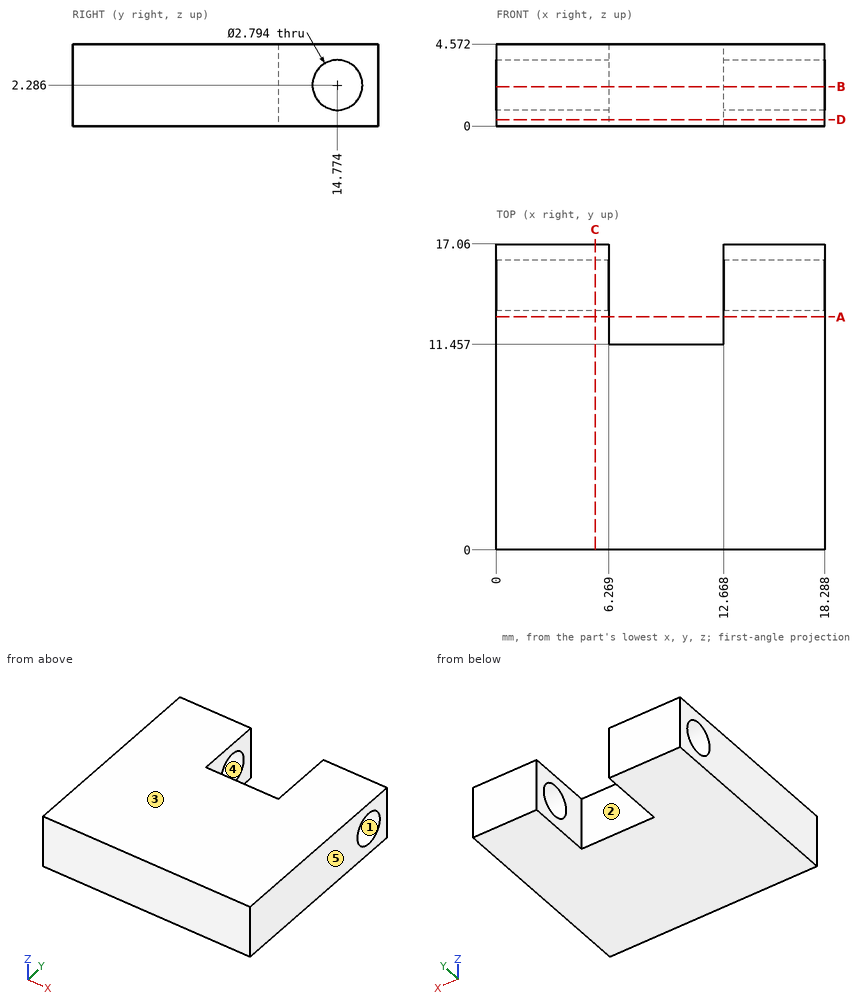
Check sheet for the drawn part. Datum: minimum x, y, z corner. Units: mm. A direction names the side the tool comes from. Coordinates: 2 decimals unless noted, no trailing zeros. Order: outer loops, then holes, each group sorted by start corner. A loop starts at its lowest first (then second) coordinate and runs counter-clockwise, first axis right, second up. Notation, with made-up numbers: (80, -32.75) -> (113, -32.75) arc R22 cw to (113, -5.75) -> close; hole circle Ø11 at (58.5, 29). An arc over 180 degrees is marked (long way). Use a Markdown table: item, result. Add a question column.
1. Cross-section at D-D (z = 0.35). Enter the section's corners in (x, y).
2. Mould release check, pull along Z, two halves, no side actions. Record for the marked faces 3, 4 and 5: pulls with the +Z half, pulls with the -Z half, needs draft (parallel to the pull), parting line crosses it, or undercut.
3. Cross-section at C-C (x = 5.5). Enter the section's corners in (y, z).
4. Set-up check for the marked faces 1 and 2: record each of +Z, -Z, +X, -X, +Y, -Y from which the full face is reachable in a straight line by a thin tool's end or side.
5. Material ranges on L1, parallel to X at y = 12.25, z = 3.95; L2, parallel to Y at x = 12.5, z = 4.1; L3, parallel to Y at x = 13, z = 1.65, recorded low to high.
6. Cross-section at A-A (y = 13). Enter the section's corners in (x, z).
7. Cross-section at B-B (z = 2.2). Enter the section's corners in (x, y), and give its area (3 significant figures).
8. Go/stop test with a flat-tipped pin: pin 1 Ø1.4 at (x, z) = (9.5, 3) entering from +Y. Record where the tip stops, or that it passes through.
Filled sheet:
| question | item | result |
|---|---|---|
| 1 | outline | (0, 0) -> (18.29, 0) -> (18.29, 17.06) -> (12.67, 17.06) -> (12.67, 11.46) -> (6.27, 11.46) -> (6.27, 17.06) -> (0, 17.06) -> close |
| 2 | face 3 | pulls with the +Z half |
| 2 | face 4 | undercut |
| 2 | face 5 | needs draft |
| 3 | outline | (0, 0) -> (17.06, 0) -> (17.06, 4.57) -> (0, 4.57) -> close; hole circle Ø2.79 at (14.77, 2.29) |
| 4 | face 1 | +X, -X |
| 4 | face 2 | +Z, -Z, +Y |
| 5 | L1 | 0 to 6.27, 12.67 to 18.29 |
| 5 | L2 | 0 to 11.46 |
| 5 | L3 | 0 to 13.53, 16.02 to 17.06 |
| 6 | outline | (0, 0) -> (6.27, 0) -> (6.27, 4.57) -> (0, 4.57) -> close; (12.67, 0) -> (18.29, 0) -> (18.29, 4.57) -> (12.67, 4.57) -> close |
| 7 | outline | (0, 0) -> (18.29, 0) -> (18.29, 13.38) -> (12.67, 13.38) -> (12.67, 11.46) -> (6.27, 11.46) -> (6.27, 13.38) -> (0, 13.38) -> close; (0, 16.17) -> (6.27, 16.17) -> (6.27, 17.06) -> (0, 17.06) -> close; (12.67, 16.17) -> (18.29, 16.17) -> (18.29, 17.06) -> (12.67, 17.06) -> close |
| 7 | area | 243 mm2 |
| 8 | pin 1 | y = 11.46 |
